Here's how the part is built. I have some questions about the finished solid (model axes, mm). A direction names the side the tool comes from. Give positions to 0.01 mm unless a question says otherwise; leave off trailing zeros. Write each loop counter-clockwise with the first axis right and the second up, starting at its lowest first coordinate (ties: lowest second). Pieces come first, ordered by that corner, then holes. Notation, with made-up numbers: (9.5, 15.25) - (13.5, 15.25) arc R11 cw to (13.5, 19.25) - close; hole circle Ø11 at (60.25, 18). An arc over 180 degrees is marked (long way). One line per item, written item: value. Start each with the question number.
1) Imagine slicing it at A-A on y = 7. Write out the boundary of the cut face in (x, z).
2) I'm going to push flat-ended pins straight in: P1, Ø0.6, axis at y = -0.5, z = 1, coming from the -X side; P2, Ø1, axis at y = 3, z = 1.5, coming from the +X side; P3, Ø1, axis at x = 2.5, z = 0.5, coming from the +Y side; P4, Ø1.5, axis at x = -2.5, y = 3.5, coming from the +Z side. Where does each tip first touch, or does it pass through?
3) Please list where these lines run through material, in increasing order: L1, parallel to X at y = 5, z = 1; L2, parallel to X at y = 5.5, z = 0.2; L3, parallel to Y at x = -6.75, z = 0.6. Write a range as [from, to].
4) We'd pull the mould along Y, two halves only. Please class faces 1 (the flat face through (-5.252, -1, 1)), 2 (the cylindrical face through (-5.013, 2.139, 0.986)), 3 (the flat face through (6.45, 1.89, 1.01)): +Y half, -Y half, draft (parallel to the pull), parting line (faces both ways), or undercut.
5) Imagine slicing it at B-B on x = -6.75. Write out the boundary of the cut face in (y, z).
6) Imagine slicing it at C-C on z = 0.5. Write out the boundary of the cut face in (x, y).
7) Imagine slicing it at D-D on y = 0.5. Write out the boundary of the cut face in (x, z), plus the area to 3 significant figures.
8) On a 3-axis mill with a long thin cutter (end or side, diameter ignored), from which of +Z, -Z, +X, -X, +Y, -Y can I reach the whole of each face in a straight line? I mean faces 4 (the flat face through (4.156, 6.903, 0.986)), 5 (the cylindrical face through (-8.365, 7.629, 0.986)), 6 (the flat face through (2, 7.984, 1)). Say none if no direction works.
Autodesk Inventor part; units mm, degrees
ref_plane "YZ Plane" through (0, 0, 0) normal (1, 0, 0) x (0, 1, 0)
ref_plane "XZ Plane" through (0, 0, 0) normal (0, 1, 0) x (-1, 0, 0)
ref_plane "XY Plane" through (0, 0, 0) normal (0, 0, 1) x (1, 0, 0)
sketch "Skizze1" plane through (0, 0, 0) normal (0, 0, 1) x (1, 0, 0)
  line L0 (-0.1001, 7.9841) -> (4.7481, 7.9841)
  line L1 (5.2519, 4.8576) -> (5.2519, 0)
  line L2 (5.2519, 0) -> (-5.2519, 0)
  line L3 (-5.2519, 0) -> (-5.2519, 0.1317)
  line L4 (0, 14.3325) -> (0, -2.5319)
  line L5 (-14.2928, 0) -> (8.5093, 0)
  line L6 (4.7481, 7.9841) -> (3.547, 5.7916)
  line L7 (3.547, 5.7916) -> (5.2519, 4.8576)
  arc A0 (-0.1001, 7.9841) -> (-5.2519, 0.1317) centre (-4.112, 5) ccw
  point P0 (0, 0)
  dimension "d34" = 8
  dimension "d36" = 2.5
  dimension "d40" = 10
  dimension "d41" = 61.286
  dimension "d42" = 5.2519
  dimension "d43" = 7.9841
  dimension "d44" = 0.1002
extrude "Extrusion2" add sketch "Skizze1" along normal blind 2
sketch "Skizze4" plane through (0, 0, 2) normal (0, 0, 1) x (1, 0, 0)
  arc A0 (-0.1001, 7.9841) -> (-5.2519, 0.1317) centre (-4.112, 5) ccw
  point P0 (0, 0)
hole "Bohrung2" at (-4.112, 5, 2) direction (0, 0, -1) diameter 6 end through all
sketch "Skizze5" plane through (-5.2519, 0, 0) normal (0, -1, 0) x (1, 0, 0)
  line L0 (0, 0) -> (10.5038, 0)
  line L1 (10.5038, 0) -> (10.5038, 2)
  line L2 (0, 2) -> (10.5038, 2)
  line L3 (0, 0) -> (0, 2)
  point P0 (5.2519, 0)
extrude "Extrusion3" add sketch "Skizze5" along normal blind 2
sketch "Skizze6" plane through (5.2519, 4.8576, 2) normal (1, 0, 0) x (0, 0, -1)
  line L0 (2, 0) -> (2, -6.8576)
  line L1 (2, 0) -> (0, 0)
  line L2 (0, 0) -> (0, -6.8576)
  line L3 (2, -6.8576) -> (0, -6.8576)
  point P0 (2, -4.8576)
extrude "Extrusion4" add sketch "Skizze6" along normal blind 2
sketch "Skizze7" plane through (0, 0, 2) normal (0, 0, 1) x (1, 0, 0)
  line L0 (-5.2519, -2) -> (7.2519, -2)
  line L1 (7.2519, 4.8576) -> (7.2519, -2)
  line L2 (-5.2519, -2) -> (7.2519, 0.7766)
  line L3 (-5.2519, -2) -> (7.5565, -2) construction
  point P0 (0, 0)
  dimension "d56" = 12.52
extrude "Extrusion5" cut sketch "Skizze7" against normal blind 2
sketch "Skizze8" plane through (-5.2519, -2, 0) normal (0.2168, -0.9762, 0) x (0.9762, 0.2168, 0)
  line L0 (0, 2) -> (12.8083, 2)
  line L1 (0, 2) -> (0, 0)
  line L2 (12.8083, 0) -> (0, 0)
  line L3 (12.8083, 2) -> (12.8083, 0)
  point P0 (5.5605, 0)
extrude "Extrusion6" add sketch "Skizze8" along normal blind 1.98
sketch "Skizze9" plane through (0, 0, 2) normal (0, 0, 1) x (1, 0, 0)
  line L0 (7.2519, 4.8576) -> (7.2519, 0.7766)
  line L1 (5.2519, 4.8576) -> (7.2519, 4.8576)
  line L2 (7.6811, -1.1563) -> (-4.8227, -3.9329)
  line L3 (7.2519, 0.7766) -> (7.6811, -1.1563)
  line L4 (5.2519, 4.8576) -> (7.6811, -1.1563)
  point P0 (0, 0)
extrude "Extrusion7" cut sketch "Skizze9" against normal blind 2
properties part number "Kontakt" material "2.0265 CuZn30(Bronze/weich)"
Numbers:
1. outline: (-8.69, 0) - (-6.35, 0) - (-6.35, 2) - (-8.69, 2) - close; (-1.88, 0) - (4.21, 0) - (4.21, 2) - (-1.88, 2) - close
2. P1: x = -5.25
2. P2: x = 6.2
2. P3: y = 7.98
2. P4: through
3. L1: [-9.11, -7.11], [-1.11, 4.99]
3. L2: [-9.09, -7.07], [-1.15, 4.08]
3. L3: [0.75, 3.57], [6.43, 9.25]
4. face 1: draft
4. face 2: undercut
4. face 3: +Y half
5. outline: (0.75, 0) - (3.57, 0) - (3.57, 2) - (0.75, 2) - close; (6.43, 0) - (9.25, 0) - (9.25, 2) - (6.43, 2) - close
6. outline: (-5.25, -2) - (-4.82, -3.93) - (7.68, -1.16) - (5.25, 4.86) - (3.55, 5.79) - (4.75, 7.98) - (-0.1, 7.98) arc R5 ccw (long way) to (-5.25, 0.13) - close; hole circle Ø6 at (-4.11, 5)
7. outline: (-6.29, 0) - (7.01, 0) - (7.01, 2) - (-6.29, 2) - close
7. area: 26.6 mm^2
8. face 4: +Z, -Z, +X
8. face 5: +Z, -Z
8. face 6: +Z, -Z, +X, +Y
